from build123d import *

# Parameters (mm, degrees)
BOSS_EXTRUDE1_DEPTH = 304.8
FILLET1_R           = 0.254
CUT_EXTRUDE1_DEPTH  = 248.9375


with BuildPart() as part:
    # Sketch3 → Boss-Extrude1 (new, symmetric)
    with BuildSketch(Plane.XY):
        Polygon((1.5875, 25.4), (0, 25.4), (0, 0), (25.4, 0), (25.4, 1.5875), (1.5875, 1.5875), align=None)
    extrude(amount=BOSS_EXTRUDE1_DEPTH, both=True)

    # Fillet1
    fillet1_edges = [part.edges().sort_by_distance(p)[0] for p in [
        (1.5875, 1.5875, 0),
    ]]
    fillet(fillet1_edges, radius=FILLET1_R)

    # Sketch4 → Cut-Extrude1 (cut)
    with BuildSketch(Plane(origin=(0, 0, -304.8), x_dir=(-1, 0, 0), z_dir=(0, 0, -1))):
        with BuildLine():
            Line((-1.5875, 25.4), (-1.5875, 1.8415))
            ThreePointArc((-1.5875, 1.8415), (-1.661894878, 1.661894878), (-1.8415, 1.5875))
            Line((-1.8415, 1.5875), (-25.4, 1.5875))
            Line((-25.4, 1.5875), (-25.4, 0))
            Line((-25.4, 0), (0, 0))
            Line((0, 0), (0, 25.4))
            Line((0, 25.4), (-1.5875, 25.4))
        make_face()
    extrude(amount=-CUT_EXTRUDE1_DEPTH, mode=Mode.SUBTRACT)


solid = part.part
Source: CAD feature listing. Evaluate the final solid. Frame: model axes, mm. A direction names the side the tool comes from. Coordinates: 2 decimals unless noted, no trailing zeros. Loops run counter-clockwise (first coordinate to the right, second up) from the corner with the lowest first, then second, coordinate; pieces in that order, holes last. Notation, with made-up numbers: (2.25, 6) -> (52.25, 6) arc R18 ccw to (52.25, 21) -> close; hole circle Ø5 at (72, -16). An arc over 180 degrees is marked (long way). Answer in a Markdown table with one row per item. Add a question column.
Q1. Ray query, line 1 along X through (y, z) = (20.5, 206.5). Return the intervals inside material, ascending.
Q2. Contact query for flat-ended pins moving along their axis: pin 1 Ø7 at (x, z) = (16.5, 198) entering from +Y; pin 2 Ø7 at (y, z) = (11.5, 183.5) entering from +X; pin 3 Ø1.5 at (x, y) = (8, 4) entering from -Z. Output: stop coordinate, or through.
Q3. Section A-A on z = 172. Return the cut outline in (x, y), and give its area (3 significant figures).
Q4. Reachability of faces 1 (the face through (1, 7, 304.8)), 2 (the face through (14, 1.588, 127)) from +Z, -Z, +X, -X, +Y, -Y: full face, straight path, thin tool, end or side. Return the list, or none.
Q5. Section B-B on y = 6.5. Return the cut outline in (x, z), and give its area (3 significant figures).
Computed values:
| question | item | result |
|---|---|---|
| 1 | line 1 | x = 0 to 1.59 |
| 2 | pin 1 | stops at y = 1.59 |
| 2 | pin 2 | stops at x = 1.59 |
| 2 | pin 3 | passes through |
| 3 | outline | (0, 0) -> (25.4, 0) -> (25.4, 1.59) -> (1.84, 1.59) arc R0.25 cw to (1.59, 1.84) -> (1.59, 25.4) -> (0, 25.4) -> close |
| 3 | area | 78.1 mm^2 |
| 4 | face 1 | +Z, +X, -X, +Y, -Y |
| 4 | face 2 | +Z, -Z, +X, +Y |
| 5 | outline | (0, -55.86) -> (1.59, -55.86) -> (1.59, 304.8) -> (0, 304.8) -> close |
| 5 | area | 573 mm^2 |
